The model under review builds one solid part; all positions refer to its coordinate system, in mm. Face numbers are marked on the shaded views. A direction names the side the tool comes from. Round coordinates to 2 decimals unless told otherwise and drop trailing zeros. Loops run counter-clockwise (first coordinate to the right, second up) from the corner with the lowest first, then second, coordinate; pieces in that order, holes last. Notation, with made-up numbers: (-33.75, 3) -> (20.25, 3) arc R20 ccw to (20.25, 35) -> close; hole circle Ø5 at (34.5, 2.5). An arc over 180 degrees is marked (long way). Use CSV: the item, a comma, the result in double quotes. Start each with the question number.
```python
from build123d import *

# Parameters (mm, degrees)
F1_DEPTH = 10
F2_R     = 2


with BuildPart() as f1:
    # F0 (on Front) → F1 (new body)
    with BuildSketch(Plane.XZ):
        Polygon((0, 26.158135), (-15, 26.317666), (-15, 6.317666), (-28.478333, 6.317666), (-28.478333, -8.682334), (-13.478333, -8.682334), (-13.478333, -43.682334), (0, -43.682334), (0, -8.841865), (15, -8.841865), (15, 6.158135), (0, 6.158135), align=None)
    extrude(amount=F1_DEPTH)

    # F2
    f2_edges = [f1.edges().sort_by_distance(p)[0] for p in [
        (-7.5, -10, 26.237901),
        (-15, -10, 16.317666),
        (-21.739167, -10, 6.317666),
        (-28.478333, -10, -1.182334),
        (-20.978333, -10, -8.682334),
        (-13.478333, -10, -26.182334),
        (-6.739167, -10, -43.682334),
        (0, -10, -26.262099),
        (7.5, -10, -8.841865),
        (15, -10, -1.341865),
        (7.5, -10, 6.158135),
        (0, -10, 16.158135),
    ]]
    fillet(f2_edges, radius=F2_R)


solid = f1.part
```
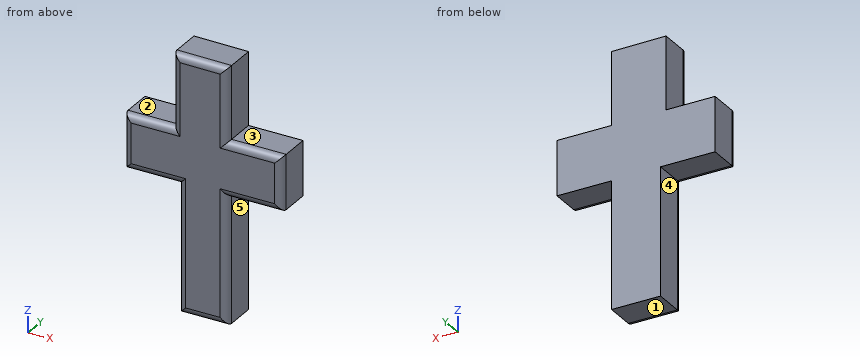
1. Take a section at B-B, the plane z = -33. Give the boundary of the cut face in (x, y), then the cut area to 3 significant figures.
2. For the marked faces 1, 2, 3, 4 and 5, list the 3-axis set-ups (+Z, -Z, +X, -X, +Y, -Y) from which the entire face can be reached by the end or side of a thin tool; tool diameter is ignored.
3. Take a section at A-A, the plane y = -1.5. Give the boundary of the cut face in (x, z), then the cut area to 3 significant figures.
4. Clearance check with flat-ended pins moving along their axes: P1, Ø1.5, axis at x = -0.5, z = -18, coming from the -Y side; P2, Ø4, axis at x = 10, y = -5.5, coming from the +Z side; P3, Ø1.5, axis at x = 9.5, y = -2.5, coming from the -Z side. State where each tip first meets the part, or that it passes through.
5. For line 1 along X through (y, z) = (-3, -26.5); line 2 along Z through (x, y) = (10, -6.75); line 3 along X through (y, z) = (-5, 14), list the stretches that pass through material, from the lowest coordinate up. Write a range as from..to.
6. Take a section at C-C, the plane x = 12. Give the boundary of the cut face in (y, z).
Results:
1,outline,"(-13.48, -8) arc R2 ccw to (-11.48, -10) -> (-2, -10) arc R2 ccw to (0, -8) -> (0, 0) -> (-13.48, 0) -> close"
1,area,"133 mm²"
2,face 1,"-Z, +X, -X, +Y, -Y"
2,face 2,"+Z, -X, +Y, -Y"
2,face 3,"+Z, +X, +Y, -Y"
2,face 4,"-Z, -X, +Y, -Y"
2,face 5,"-Z, +X, +Y, -Y"
3,outline,"(-28.48, -8.68) -> (-13.48, -8.68) -> (-13.48, -43.68) -> (0, -43.68) -> (0, -8.84) -> (15, -8.84) -> (15, 6.16) -> (0, 6.16) -> (0, 26.16) -> (-15, 26.32) -> (-15, 6.32) -> (-28.48, 6.32) -> close"
3,area,"1,420 mm²"
4,P1,"y = -9.85"
4,P2,"z = 6.16"
4,P3,"z = -8.84"
5,line 1,"-13.48..0"
5,line 2,"-8.84..6.16"
5,line 3,"-15..0"
6,outline,"(-10, -6.84) arc R2 ccw to (-8, -8.84) -> (0, -8.84) -> (0, 6.16) -> (-8, 6.16) arc R2 ccw to (-10, 4.16) -> close"
